from build123d import *

# Parameters (mm, degrees)
F0_R        = 2.5
F1_DEPTH    = 10
F2_W        = 8.8
F2_H        = 8.8
F2_R        = 2.5
F3_DEPTH    = 2.5
F4_W        = 8.8
F4_H        = 8.8
F4_R        = 2.5
F5_DEPTH    = 2.5
F6_T1_DEPTH = 52.7272001401
F6_T3_DEPTH = 37.6344553761
F6_T5_DEPTH = 42.8447953281
F6_T7_DEPTH = 58.0308217405
F6_T9_DEPTH = 38.1595084339
F7_T1_DEPTH = 58.883894651


# Not quite as in the source:
# - a fillet or chamfer that OpenCascade refuses, or shapes differently, is made with other operations: its cross-section is extruded or revolved along the edge and cut away or added


with BuildPart() as f1:
    # F0 (on Top) → F1 (new body)
    with BuildSketch(Plane.XY):
        Polygon((10.7213496009, 14.3520427298), (0, 14.3520427298), (-6.0058505391, 14.3520427298), (-6.0058505391, 11.3520427298), (-14.8058505391, 11.3520427298), (-14.8058505391, 2.5520427298), (-6.0058505391, 2.5520427298), (-6.0058505391, -1.4479572702), (0, -1.4479572702), (16.0249712014, -1.4479572702), (22.5786776848, 0.5269235903), (25.5761091025, 2.9657761595), (26.8709543148, 4.6940274585), (27.0316003021, 7.267983998), (27.0316003021, 9.1232445721), (26.8709543148, 10.7497860696), (25.5761091025, 12.8667177236), (24.1809434093, 13.3803505253), (25.5761091025, 14.2337194165), (13.9262006316, 13.0831117922), align=None)
        with Locations((-10.4058505391, 6.9520427298)):
            Circle(F0_R, mode=Mode.SUBTRACT)
    extrude(amount=F1_DEPTH)

    # F2 (on face) → F3 (cut)
    with BuildSketch(Plane.XY.offset(10)):
        with Locations((-10.4058505391, 6.9520427298)):
            Rectangle(F2_W, F2_H)
        with Locations((-10.4058505391, 6.9520427298)):
            Circle(F2_R, mode=Mode.SUBTRACT)
    extrude(amount=-F3_DEPTH, mode=Mode.SUBTRACT)

    # F4 (on face) → F5 (cut)
    with BuildSketch(Plane(origin=(0, 0, 0), x_dir=(1, 0, 0), z_dir=(0, 0, -1))):
        with Locations((-10.4058505391, -6.9520427298)):
            Rectangle(F4_W, F4_H)
        with Locations((-10.4058505391, -6.9520427298)):
            Circle(F4_R, mode=Mode.SUBTRACT)
    extrude(amount=-F5_DEPTH, mode=Mode.SUBTRACT)

    # F6: fillet of radius 3 on 5 edges, made by hand

    # F6_s2 → F6_t1 (cut)
    with BuildSketch(Plane.YZ.offset(-24.0058505391)):
        with BuildLine():
            ThreePointArc((14.3520427298, 3), (13.4733630734, 0.8786796564), (11.3520427298, 0))
            Line((11.3520427298, 0), (11.3520427298, -0.06))
            Line((11.3520427298, -0.06), (14.4120427298, -0.06))
            Line((14.4120427298, -0.06), (14.4120427298, 3))
            Line((14.4120427298, 3), (14.3520427298, 3))
        make_face()
    extrude(amount=F6_T1_DEPTH, mode=Mode.SUBTRACT)

    # F6_s4 → F6_t3 (cut)
    with BuildSketch(Plane(origin=(1.1379480439, -11.5217301503, 0), x_dir=(0, 0, 1), z_dir=(-0.0982871663, 0.9951580944, 0))):
        with BuildLine():
            ThreePointArc((0, 24.7974137027), (0.8786796564, 26.9187340462), (3, 27.7974137027))
            Line((3, 27.7974137027), (3, 27.8574137027))
            Line((3, 27.8574137027), (-0.06, 27.8574137027))
            Line((-0.06, 27.8574137027), (-0.06, 24.7974137027))
            Line((-0.06, 24.7974137027), (0, 24.7974137027))
        make_face()
    extrude(amount=F6_T3_DEPTH, mode=Mode.SUBTRACT)

    # F6_s6 → F6_t5 (cut)
    with BuildSketch(Plane(origin=(-2.9435517348, -0.8870040179, 0), x_dir=(0, 0, 1), z_dir=(0.9574729658, 0.2885229968, 0))):
        with BuildLine():
            ThreePointArc((0, 3.0099526564), (0.8786796564, 5.131273), (3, 6.0099526564))
            Line((3, 6.0099526564), (3, 6.0699526564))
            Line((3, 6.0699526564), (-0.06, 6.0699526564))
            Line((-0.06, 6.0699526564), (-0.06, 3.0099526564))
            Line((-0.06, 3.0099526564), (0, 3.0099526564))
        make_face()
    extrude(amount=F6_T5_DEPTH, mode=Mode.SUBTRACT)

    # F6_s8 → F6_t7 (cut)
    with BuildSketch(Plane.YZ.offset(-24.0058505391)):
        with BuildLine():
            ThreePointArc((1.5520427298, 0), (-0.5692776137, 0.8786796564), (-1.4479572702, 3))
            Line((-1.4479572702, 3), (-1.5079572702, 3))
            Line((-1.5079572702, 3), (-1.5079572702, -0.06))
            Line((-1.5079572702, -0.06), (1.5520427298, -0.06))
            Line((1.5520427298, -0.06), (1.5520427298, 0))
        make_face()
    extrude(amount=F6_T7_DEPTH, mode=Mode.SUBTRACT)

    # F6_s10 → F6_t9 (cut)
    with BuildSketch(Plane(origin=(-0.1744913342, -0.2328964668, 0), x_dir=(0, 0, 1), z_dir=(0.5996018316, 0.8002984715, 0))):
        with BuildLine():
            ThreePointArc((0, 15.6902362056), (0.8786796564, 17.8115565491), (3, 18.6902362056))
            Line((3, 18.6902362056), (3, 18.7502362056))
            Line((3, 18.7502362056), (-0.06, 18.7502362056))
            Line((-0.06, 18.7502362056), (-0.06, 15.6902362056))
            Line((-0.06, 15.6902362056), (0, 15.6902362056))
        make_face()
    extrude(amount=F6_T9_DEPTH, mode=Mode.SUBTRACT)

    # F7: chamfer of 10 x 3.6397023427 on 1 edges, made by hand

    # F7_s2 → F7_t1 (cut)
    with BuildSketch(Plane.XY.offset(-22.9419473255)):
        Polygon((-6.0058505391, 2.1917450725), (3.9941494609, -1.4479572702), (-6.0058505391, -1.4479572702), align=None)
    extrude(amount=F7_T1_DEPTH, mode=Mode.SUBTRACT)


solid = f1.part
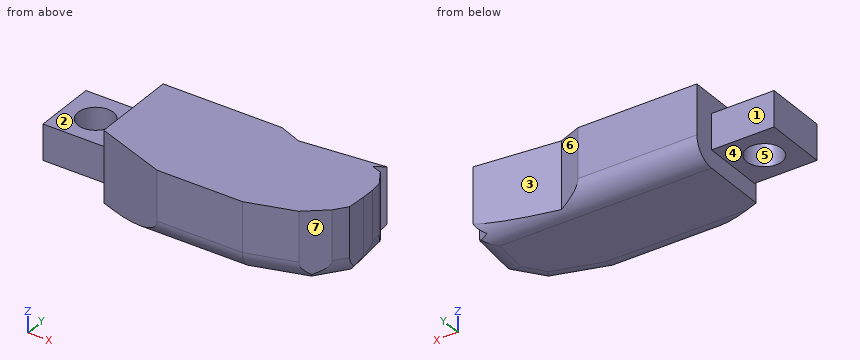
CAD build for the part. Positions are in the model's coordinates, mm. Face numbers are marked on the shaded views. A direction names the side the tool comes from. Give positions to 0.01 mm unless a question says otherwise; leave off trailing zeros. Loops run counter-clockwise (first coordinate to the right, second up) from the corner with the lowest first, then second, coordinate; pieces in that order, holes last. Notation, with made-up numbers: M 55,66 L 82,66 A22 cw 82,95 Z; hole C 19.25,4.25 d11. An arc over 180 degrees is marked long. Answer in a Markdown table with one row per item. Add a question column.
Item 1: Band-saw the part on B-B on x = 6.5. Give the cut face in (y, z).
Item 2: Mould opens along Y. For the marked faces 5, 6 and 7 say: +Y half, -Y half, draft (parallel to the pull), parting line (faces both ways), or undercut.
Item 3: Drop flat-ended pins along their axis: P1, Ø2, axis at x = -7.5, y = 6.5, coming from the -Z side; P2, Ø4.5, axis at x = -12, y = 9, coming from the +Z side; P3, Ø1.5, axis at y = 2, z = 1, coming from the -X side. Give the stop position or say it passes through.
Item 4: Band-saw the part on A-A on z = 8.25. Give the cut face in (x, y), then the cut area to 3 significant figures.
Item 5: Probe probe 1 along X at (y, z) = (3.25, 2); probe 2 along Y at (x, z) = (-10, 4); probe 3 along X at (y, z) = (7.75, 8.75). List the from-to ranges inside material, lowest first.
Item 6: Band-saw the part on C-C on x = -1.5. Give the cut face in (y, z).
Item 7: Tool access for the marked faces 1, 2, 3 and 4: list every direction of +Z, -Z, +X, -X, +Y, -Y with a clear straight run to the whole face (end or side of a thin tool).
Reply:
| question | item | result |
|---|---|---|
| 1 | outline | M -1.45,3 A3 ccw 1.55,0 L 11.35,0 A3 ccw 14.35,3 L 14.35,10 L -1.45,10 Z |
| 2 | face 5 | undercut |
| 2 | face 6 | +Y half |
| 2 | face 7 | -Y half |
| 3 | P1 | stops at z = 2.5 |
| 3 | P2 | stops at z = 7.5 |
| 3 | P3 | stops at x = -6.01 |
| 4 | outline | M -6.01,2.19 L 3.99,-1.45 L 16.02,-1.45 L 22.58,0.53 L 25.58,2.97 L 26.87,4.69 L 27.03,7.27 L 27.03,9.12 L 26.87,10.75 L 25.58,12.87 L 24.18,13.38 L 25.58,14.23 L 13.93,13.08 L 10.72,14.35 L -6.01,14.35 Z |
| 4 | area | 465 mm^2 |
| 5 | probe 1 | x = -6.01 to 25.57 |
| 5 | probe 2 | y = 2.55 to 4.49, 9.42 to 11.35 |
| 5 | probe 3 | x = -6.01 to 27.03 |
| 6 | outline | M 0.55,0.17 A3 ccw 1.55,0 L 11.35,0 A3 ccw 14.35,3 L 14.35,10 L 0.55,10 Z |
| 7 | face 1 | +Z, -Z, -X, +Y |
| 7 | face 2 | +Z, -X, +Y, -Y |
| 7 | face 3 | +Z, -Z, +Y |
| 7 | face 4 | -Z, -X, +Y, -Y |
